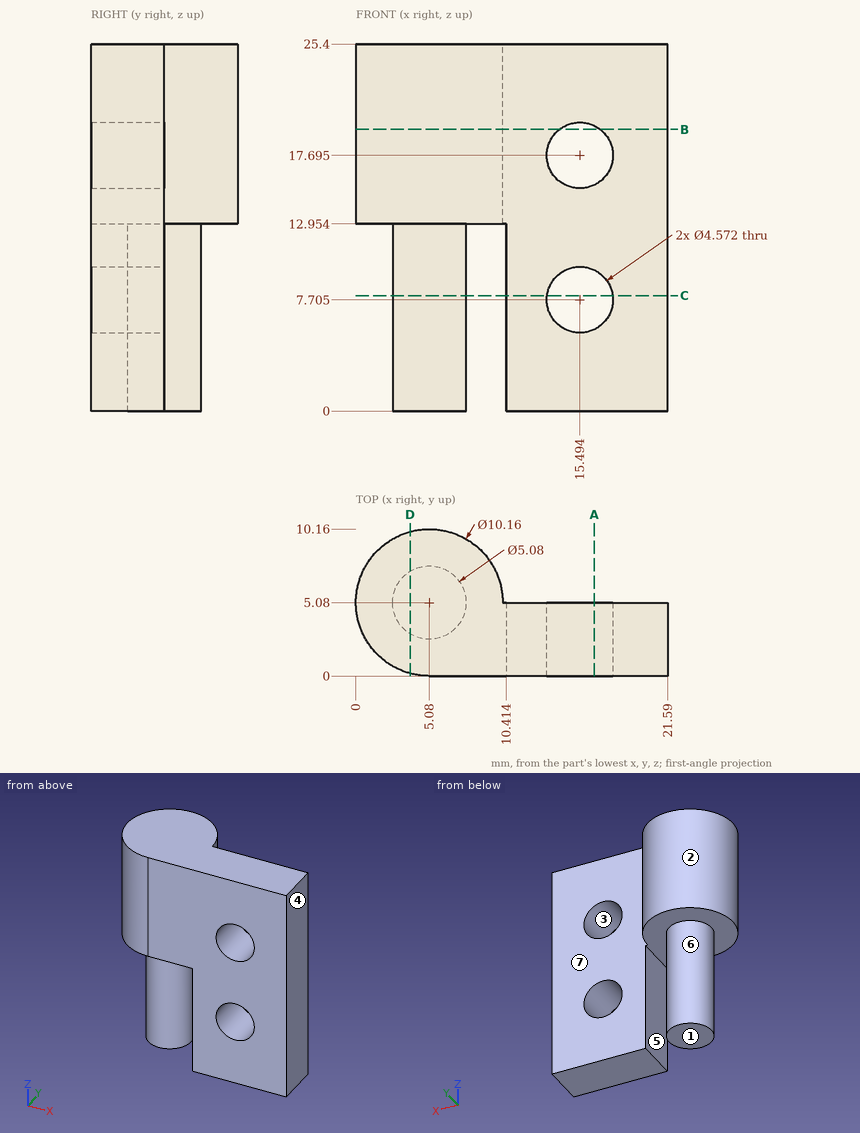
Can you work these out from the drawing? Everything is in mm from the part's minimum corner. A direction names the side the tool comes from. Give positions to 0.01 mm unless a question says otherwise; leave off trailing zeros. Loops run counter-clockwise (first coordinate to the right, second up) from the corner with the lowest first, then second, coordinate; pieces in that order, holes last. Notation, with made-up numbers: M 12,52.5 L 26,52.5 A35 ccw 26,84.5 Z; hole C -3,-13 d1. An arc over 180 degrees is marked long. Put each result on its own line as item: value. Start each with the question number.
(1) I need wall thicknesses on line 1 along Z through (x, y) = (14.75, 3.5); line 2 along X through (y, z) = (4, 19.5) (1 decimal); line 3 along Y through (x, z) = (20, 2). Which ranges of each line are inside material? Lowest first, please. Write a range as [from, to].
(2) I want a section at A-A on x = 16.5. Please give me the cut outline in (y, z).
(3) I want a section at C-C on z = 8. Please give me the cut outline in (x, y).
(4) If we mould it in two halves opening along Z, with no side actions, what happens to the marked faces 1, 2 and 3? For each: +Z half, -Z half, draft (parallel to the pull), parting line (faces both ways), or undercut.
(5) I want a section at D-D on x = 3.75. Please give me the cut outline in (y, z), then the cut area to 3 significant figures.
(6) Will these pins go through, and if not, where does the flat tip stop? pin 1 Ø1.5 at (y, z) = (2, 7) entering from -X; pin 2 Ø1 at (y, z) = (3.5, 6.5) entering from -X; pin 3 Ø12.5 at (x, z) = (18.5, 16.5) entering from +Y.
(7) I want a section at B-B on z = 19.5. Please give me the cut outline in (x, y).
(8) For the marked faces 4, 5, 6 and 7, which set-ups out of +Z, -Z, +X, -X, +Y, -Y let a thin tool reach every point of the face, with its end or its side?
Answer block:
1. line 1: [0, 5.54], [9.87, 15.53], [19.86, 25.4]
1. line 2: [0.1, 14.1], [16.9, 21.6]
1. line 3: [0, 5.08]
2. outline: M 0,0 L 5.08,0 L 5.08,5.65 L 0,5.65 Z; M 0,9.76 L 5.08,9.76 L 5.08,15.64 L 0,15.64 Z; M 0,19.75 L 5.08,19.75 L 5.08,25.4 L 0,25.4 Z
3. outline: C 5.08,5.08 d5.08; M 10.41,0 L 13.23,0 L 13.23,5.08 L 10.41,5.08 Z; M 17.76,0 L 21.59,0 L 21.59,5.08 L 17.76,5.08 Z
4. face 1: -Z half
4. face 2: draft
4. face 3: undercut
5. outline: M 0.18,12.95 L 2.92,12.95 L 2.92,0 L 7.24,0 L 7.24,12.95 L 9.98,12.95 L 9.98,25.4 L 0.18,25.4 Z
5. area: 178 mm^2
6. pin 1: x = 4.07
6. pin 2: x = 2.78
6. pin 3: y = 5.08
7. outline: M 5.08,0 L 14.09,0 L 14.09,5.08 L 10.16,5.08 A5.08 ccw long Z; M 16.9,0 L 21.59,0 L 21.59,5.08 L 16.9,5.08 Z
8. face 4: +Z, -Z, +X, +Y, -Y
8. face 5: -Z, +Y, -Y
8. face 6: -Z
8. face 7: +Z, -Z, +X, +Y
